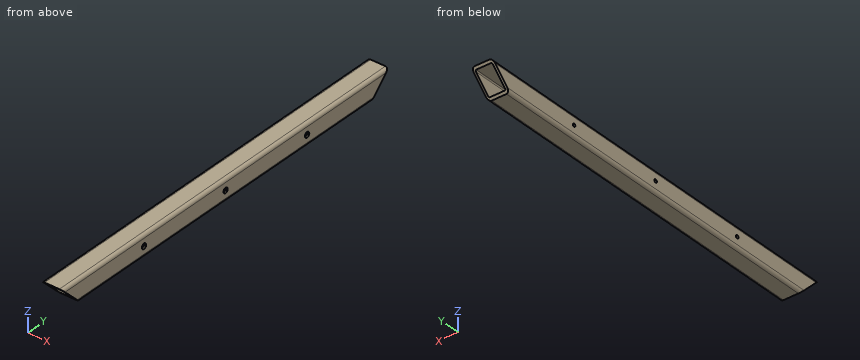
from build123d import *

# Parameters (mm, degrees)
F2_W            = 20
F2_H            = 20
F3_DEPTH        = 190
F4_R            = 3
F5_T            = -2
F7_DEPTH        = 20.001
F9_DEPTH        = 20.001
F11_D           = 3
F11_CSINK_D     = 5
F11_CSINK_ANGLE = 90


with BuildPart() as f3:
    # F2 (on Front) → F3 (new body, symmetric)
    with BuildSketch(Plane.XZ):
        Rectangle(F2_W, F2_H)
    extrude(amount=F3_DEPTH, both=True)

    # F4
    f4_edges = [f3.edges().sort_by_distance(p)[0] for p in [
        (10, 0, 10),
        (-10, 0, 10),
        (10, 0, -10),
        (-10, 0, -10),
    ]]
    fillet(f4_edges, radius=F4_R)

    # F5
    f5_openings = [f3.faces().sort_by_distance(p)[0] for p in [
        (0, -190, 0),
        (0, 190, 0),
    ]]
    offset(amount=F5_T, openings=f5_openings)

    # F6 (on face) → F7 (cut, through all)
    with BuildSketch(Plane(origin=(-10, 0, 0), x_dir=(0, -1, 0), z_dir=(-1, 0, 0))):
        Polygon((-190, 10), (-190, -10), (-170, -10), align=None)
    extrude(amount=-F7_DEPTH, mode=Mode.SUBTRACT)

    # F8 (on face) → F9 (cut, through all)
    with BuildSketch(Plane.YZ.offset(10)):
        Polygon((-190, -10), (-170, -10), (-190, 10), align=None)
    extrude(amount=-F9_DEPTH, mode=Mode.SUBTRACT)

    # F11 (through all)
    with Locations(Plane.YZ.offset(10)):
        with Locations((95, 0), (0, 0), (-95, 0)):
            CounterSinkHole(F11_D / 2, F11_CSINK_D / 2, counter_sink_angle=F11_CSINK_ANGLE)


solid = f3.part
Build history of the part. All positions in model axes, mm. Round coordinates to 2 decimals unless told otherwise and drop trailing zeros. Order: outer loops, then holes, each group sorted by start corner. A loop starts at its lowest first (then second) coordinate and runs counter-clockwise, first axis right, second up. Notation, with made-up numbers: M 49.25,-24.75 L 94.25,-24.75 A22 ccw 94.25,-6.75 Z; hole C 0.5,69.25 d6. An arc over 180 degrees is marked long. Use CSV: the item, a comma, the result in double quotes. Start each with the question number.
(1) Cut at A-A on y = -85. List the corners of the cut face in (x, z), then the cut area to 3 significant figures.
(2) Drill centre lines: probe 1 along Z at (x, y) = (5.5, 83.5); probe 2 along Y at (x, z) = (8.65, 0). Where is each one in solid material? Low to high.
(3) Flat gauge pins, fed straight in: P1, Ø2.5, axis at y = -95, z = 0, coming from the -X side; P2, Ø3.5, axis at y = 95, z = 0, coming from the +X side; P3, Ø4, axis at y = 0, z = 0, coming from the +X side. Where does each tip first touch, or does it go through?
Findings:
1,outline,"M -10,-7 A3 ccw -7,-10 L 7,-10 A3 ccw 10,-7 L 10,7 A3 ccw 7,10 L -7,10 A3 ccw -10,7 Z; hole M -8,-7 A1 ccw -7,-8 L 7,-8 A1 ccw 8,-7 L 8,7 A1 ccw 7,8 L -7,8 A1 ccw -8,7 Z"
1,area,"137 mm^2"
2,probe 1,"z = -10 to -8, 8 to 10"
2,probe 2,"y = -180 to -96.5, -93.5 to -1.5, 1.5 to 93.5, 96.5 to 180"
3,P1,"passes through"
3,P2,"stops at x = 9.25"
3,P3,"stops at x = 9.5"
